Geometry check sheet. Reference: the model listing, model coordinates, mm. Face numbers are marked on the shaded views. A direction names the side the tool comes from. Give positions to 0.01 mm unless a question says otherwise; leave off trailing zeros. Write each loop counter-clockwise with the first axis right and the second up, starting at its lowest first coordinate (ties: lowest second). Pieces come first, ordered by that corner, then holes. Notation, with made-up numbers: (23.5, -27.5) - (71.5, -27.5) arc R27 ccw to (71.5, 6.5) - close; hole circle Ø8 at (52, 77). An arc over 180 degrees is marked (long way). Use a Markdown table: item, result.
```python
from build123d import *

# Parameters (mm, degrees)
SKETCH1_W                    = 99
SKETCH1_H                    = 25
SKETCH1_W_2                  = 93
SKETCH1_H_2                  = 19
BOSS_EXTRUDE1_DEPTH          = 10
SKETCH2_R                    = 40
CUT_EXTRUDE1_DEPTH           = 8
SKETCH5_W                    = 10
SKETCH5_H                    = 25
BOSS_EXTRUDE5_DEPTH          = 2
SKETCH6_W                    = 6
SKETCH6_H                    = 19
BOSS_EXTRUDE6_DEPTH          = 2
SKETCH7_W                    = 8
SKETCH7_H                    = 3
BOSS_EXTRUDE7_DEPTH          = 30
FILLET5_R                    = 3
FILLET7_R                    = 5
FILLET8_R                    = 20
FILLET9_R                    = 1.5
FILLET10_R                   = 6
FILLET11_R                   = 3
SKETCH8_W                    = 20
SKETCH8_H                    = 25
BOSS_EXTRUDE8_DEPTH          = 2
SKETCH9_W                    = 9.8
SKETCH9_H                    = 12
BOSS_EXTRUDE9_DEPTH          = 10
SKETCH10_R                   = 2
CUT_EXTRUDE2_DEPTH           = 23
FILLET12_R                   = 6
CUT_EXTRUDE_THIN1_DEPTH      = 65.857536204
CUT_EXTRUDE_THIN1_DEPTH_BACK = 65.857536204
SKETCH11_W                   = 109.8
SKETCH11_H                   = 112
SKETCH11_W_2                 = 9.8
SKETCH11_H_2                 = 12
SKETCH12_W                   = 9.8
SKETCH12_H                   = 1
BOSS_EXTRUDE10_DEPTH         = 5


with BuildPart() as part:
    # Sketch1 → Boss-Extrude1 (new body)
    with BuildSketch(Plane(origin=(0, 0, 0), x_dir=(1, 0, 0), z_dir=(0, 1, 0))):
        Rectangle(SKETCH1_W, SKETCH1_H)
        Rectangle(SKETCH1_W_2, SKETCH1_H_2, mode=Mode.SUBTRACT)
    extrude(amount=BOSS_EXTRUDE1_DEPTH)

    # Sketch2 → Cut-Extrude1 (cut)
    with BuildSketch(Plane.XY.offset(12.5)):
        with Locations((21.780912994, 42.853113242)):
            Circle(SKETCH2_R)
    extrude(amount=-CUT_EXTRUDE1_DEPTH, mode=Mode.SUBTRACT)

    # Sketch5 → Boss-Extrude5 (add)
    with BuildSketch(Plane.XZ):
        with Locations((-29.5, 0)):
            Rectangle(SKETCH5_W, SKETCH5_H)
    extrude(amount=-BOSS_EXTRUDE5_DEPTH)

    # Sketch6 → Boss-Extrude6 (add)
    with BuildSketch(Plane.XZ):
        with Locations((43.5, 0)):
            Rectangle(SKETCH6_W, SKETCH6_H)
    extrude(amount=-BOSS_EXTRUDE6_DEPTH)

    # Sketch7 → Boss-Extrude7 (add)
    with BuildSketch(Plane(origin=(0, 10, 0), x_dir=(1, 0, 0), z_dir=(0, 1, 0))):
        with Locations((-32.5, -11)):
            Rectangle(SKETCH7_W, SKETCH7_H)
    extrude(amount=BOSS_EXTRUDE7_DEPTH)

    # Fillet5
    fillet5_edges = [part.edges().sort_by_distance(p)[0] for p in [
        (-34.5, 1, 9.5),
        (-24.5, 1, 9.5),
        (-24.5, 1, -9.5),
        (-34.5, 1, -9.5),
        (40.5, 1, -9.5),
        (40.5, 1, 9.5),
    ]]
    fillet(fillet5_edges, radius=FILLET5_R)

    # Fillet7
    fillet7_edges = [part.edges().sort_by_distance(p)[0] for p in [
        (44.599172136, 10, 11),
    ]]
    fillet(fillet7_edges, radius=FILLET7_R)

    # Fillet8
    fillet8_edges = [part.edges().sort_by_distance(p)[0] for p in [
        (-1.037346149, 10, 11),
    ]]
    fillet(fillet8_edges, radius=FILLET8_R)

    # Fillet9
    fillet9_edges = [part.edges().sort_by_distance(p)[0] for p in [
        (46.5, 6, 9.5),
        (46.5, 6, -9.5),
        (-46.5, 5, -9.5),
        (-46.5, 5, 9.5),
        (-49.5, 5, 12.5),
        (-49.5, 5, -12.5),
        (49.5, 5, -12.5),
        (49.5, 5, 12.5),
    ]]
    fillet(fillet9_edges, radius=FILLET9_R)

    # Fillet10
    fillet10_edges = [part.edges().sort_by_distance(p)[0] for p in [
        (-36.5, 10, 11),
        (-28.5, 10, 11),
    ]]
    fillet(fillet10_edges, radius=FILLET10_R)

    # Fillet11
    fillet11_edges = [part.edges().sort_by_distance(p)[0] for p in [
        (-36.5, 40, 11),
        (-28.5, 40, 11),
    ]]
    fillet(fillet11_edges, radius=FILLET11_R)

    # Sketch8 → Boss-Extrude8 (add)
    with BuildSketch(Plane.XZ):
        Rectangle(SKETCH8_W, SKETCH8_H)
    extrude(amount=-BOSS_EXTRUDE8_DEPTH)

    # Sketch9 → Boss-Extrude9 (add)
    with BuildSketch(Plane.XZ):
        Rectangle(SKETCH9_W, SKETCH9_H)
    extrude(amount=BOSS_EXTRUDE9_DEPTH)

    # Sketch10 → Cut-Extrude2 (cut)
    with BuildSketch(Plane(origin=(4.9, 0, 0), x_dir=(0, 0, -1), z_dir=(1, 0, 0))):
        with Locations((0, -5)):
            Circle(SKETCH10_R)
    extrude(amount=-CUT_EXTRUDE2_DEPTH, mode=Mode.SUBTRACT)

    # Fillet12
    fillet12_edges = [part.edges().sort_by_distance(p)[0] for p in [
        (0, -10, 6),
        (0, -10, -6),
    ]]
    fillet(fillet12_edges, radius=FILLET12_R - 0.0001)  # a hair under: the kernel refuses the full size

    # Sketch11 → Cut-Extrude-Thin1 (cut, two sides: drawn at the far end of the back side and taken through both)
    with BuildSketch(Plane.XZ.offset(-CUT_EXTRUDE_THIN1_DEPTH_BACK)):
        Rectangle(SKETCH11_W, SKETCH11_H)
        Rectangle(SKETCH11_W_2, SKETCH11_H_2, mode=Mode.SUBTRACT)
    extrude(amount=CUT_EXTRUDE_THIN1_DEPTH + CUT_EXTRUDE_THIN1_DEPTH_BACK, mode=Mode.SUBTRACT)

    # Sketch12 → Boss-Extrude10 (add)
    with BuildSketch(Plane(origin=(0, 0, -6), x_dir=(-1, 0, 0), z_dir=(0, 0, -1))):
        with Locations((0, -0.5)):
            Rectangle(SKETCH12_W, SKETCH12_H)
    boss_extrude10 = extrude(amount=BOSS_EXTRUDE10_DEPTH)

    # Mirror1: Boss-Extrude10 across plane
    add(boss_extrude10.mirror(Plane.XY))


solid = part.part
```
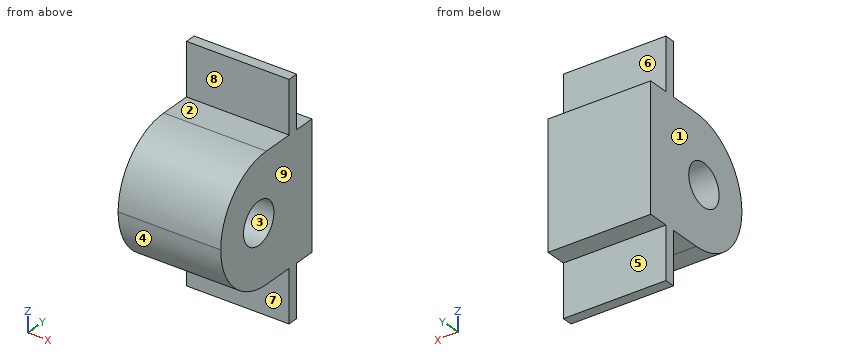
1) Depth check by flat-ended pin: P1, Ø2.5, axis at y = -5, z = 0, coming from the -X side; P2, Ø1.6, axis at x = -1.5, y = 1, coming from the -Z side; P3, Ø0.6, axis at x = -1, y = 1, coming from the +Z side; P4, Ø3.5, axis at x = -2, y = -2, coming from the +Z side. Enter the tip coordinate at first touch or a pass-through.
Working result:
| item | result |
|---|---|
| P1 | passes through |
| P2 | stops at z = -6 |
| P3 | stops at z = 6 |
| P4 | stops at z = 11 |
2) Section check D-D on y = -2. Record the boundary of the cut face in (x, z), then the cut area to 3 significant figures.
Working result:
| item | result |
|---|---|
| outline | (-4.9, -6) - (4.9, -6) - (4.9, 6) - (-4.9, 6) - close |
| area | 118 mm² |
3) Material ranges on L1, parallel to Y at x = 4.75, z = 9.5; L2, parallel to Y at x = -2.5, z = 0; L3, parallel to Z at x = -1, y = -4, recorded low to high. Write a range as from..to.
Working result:
| item | result |
|---|---|
| L1 | y = -1..0 |
| L2 | y = -10..-7, -3..2 |
| L3 | z = -6..-1.73, 1.73..6 |
4) Mould release check, pull along Z, two halves, no side actions. Record for the marked faces 1, 2, 3 and 4: pulls with the +Z half, pulls with the -Z half, needs draft (parallel to the pull), parting line crosses it, or undercut.
Working result:
| item | result |
|---|---|
| face 1 | needs draft |
| face 2 | pulls with the +Z half |
| face 3 | undercut |
| face 4 | pulls with the -Z half |
5) Section check C-C on z = -0.5. Record the boundary of the cut face in (x, y).
Working result:
| item | result |
|---|---|
| outline | (-4.9, -9.98) - (4.9, -9.98) - (4.9, -6.94) - (-4.9, -6.94) - close; (-4.9, -3.06) - (4.9, -3.06) - (4.9, 2) - (-4.9, 2) - close |
6) Section check B-B on y = -5. Record the boundary of the cut face in (x, z).
Working result:
| item | result |
|---|---|
| outline | (-4.9, -5.92) - (4.9, -5.92) - (4.9, -2) - (-4.9, -2) - close; (-4.9, 2) - (4.9, 2) - (4.9, 5.92) - (-4.9, 5.92) - close |
7) Set-up check for the marked faces 5, 6, 7, 8 and 9: record each of +Z, -Z, +X, -X, +Y, -Y from which the full face is reachable in a straight line by a thin tool's end or side.
Working result:
| item | result |
|---|---|
| face 5 | -Z, +X, -X, +Y |
| face 6 | +Z, +X, -X, +Y |
| face 7 | -Z, +X, -X, -Y |
| face 8 | +Z, +X, -X, -Y |
| face 9 | +Z, -Z, +X, +Y, -Y |
